Autodesk Inventor part; units mm, degrees
ref_plane "YZ Plane" through (0, 0, 0) normal (1, 0, 0) x (0, 1, 0)
ref_plane "XZ Plane" through (0, 0, 0) normal (0, 1, 0) x (-1, 0, 0)
ref_plane "XY Plane" through (0, 0, 0) normal (0, 0, 1) x (1, 0, 0)
sketch "Skizze1" plane through (0, 0, 0) normal (0, 1, 0) x (-1, 0, 0)
  line L0 (0, -28.6) -> (0, 10.6)
  line L1 (-14, 0) -> (14, 0)
  line L2 (-10, 5) -> (10, 5)
  line L3 (10, 5) -> (10, -5)
  line L4 (10, -5) -> (-10, -5)
  line L5 (-10, -5) -> (-10, 5)
  line L6 (-10, 5) -> (10, -5) construction
  line L7 (10, 5) -> (-10, -5) construction
  line L8 (-5, -5) -> (5, -5)
  line L9 (5, -5) -> (5, -23)
  line L10 (5, -23) -> (-5, -23)
  line L11 (-5, -23) -> (-5, -5)
  line L12 (-5, -5) -> (5, -23) construction
  line L13 (5, -5) -> (-5, -23) construction
  point P0 (0, 0)
  point P1 (0, -14)
  point P2 (-5, -5)
  point P3 (5, -5)
  dimension "d0" = 20
  dimension "d1" = 10
  dimension "d2" = 10
  dimension "d3" = 18
extrude "Extrusion1" add sketch "Skizze1" along normal blind 5
sketch "Skizze2" plane through (0, 5, 0) normal (0, 1, 0) x (1, 0, 0)
  line L0 (0, 28.6) -> (0, -10.6)
  line L1 (5, 23) -> (-5, 23)
  line L2 (-10, -5) -> (10, -5)
  point P0 (0, 0)
  point P1 (0, 17)
  dimension "d14" = 22
hole "Bohrung1" at (0, 5, -17) direction (0, -1, 0) diameter 3.4 end through all counterbore diameter 6.5 counterbore depth 3.4
sketch "Skizze3" plane through (0, 5, 0) normal (0, 1, 0) x (1, 0, 0)
  line L0 (-10, -5) -> (10, -5)
  line L1 (10, -5) -> (10, 5)
  line L2 (-10, -5) -> (10, -5)
  line L3 (10, -5) -> (10, 5)
  line L4 (10, 5) -> (-10, 5)
  line L5 (-10, 5) -> (-10, -5)
  point P0 (0, 0)
extrude "Extrusion2" add sketch "Skizze3" along normal blind 2
sketch "Skizze4" plane through (0, 0, 0) normal (0, -1, 0) x (1, 0, 0)
  line L0 (-10, 5) -> (10, 5)
  line L1 (10, -5) -> (5, -5)
  line L2 (10, 5) -> (7.75, 5)
  line L3 (7.75, 5) -> (7.75, -5)
  line L4 (7.75, -5) -> (10, -5)
  line L5 (10, -5) -> (10, 5)
  point P0 (0, 0)
  dimension "d17" = 2.25
extrude "Extrusion3" add sketch "Skizze4" along normal blind 2
mirror "Spiegeln1" about plane through (0, 0, 0) normal (1, 0, 0) of "Extrusion3"
fillet "Rundung1" radius 2 4 edges at (5, 2.5, -23) (-5, 2.5, -23) (10, 2.5, 5) (-10, 2.5, 5)
fillet "Rundung2" radius 2 2 edges at (10, 2.5, -5) (-10, 2.5, -5)
properties part number "28_Switch_Holder_Y" material "PET-Kunststoff"
Check sheet for the modelled part. Datum: model origin and axes. Units: mm. A direction names the side the tool comes from. Round coordinates to 2 decimals unless told otherwise and drop trailing zeros. Loops run counter-clockwise (first coordinate to the right, second up) from the corner with the lowest first, then second, coordinate; pieces in that order, holes last.
1. Sectioned sample at B-B on x = 0. Record the boundary of the cut face in (y, z).
2. Scan lines: probe 1 along X at (y, z) = (4, -17); probe 2 along Z at (x, y) = (0, 2.9); probe 3 along X at (y, z) = (0.85, -17). Record each from-to range of solid material in increasing order.
3. Gauge pin test, flat ends, axial feed: pin 1 Ø8 at (x, z) = (-1.5, -6) entering from -Y; pin 2 Ø3 at (x, z) = (6, -17) entering from +Y; pin 3 Ø1 at (x, z) = (-1.5, -17) entering from +Y. Record the tip position at first contact, or that the pin passes through.
4. Set-up check for faces 1 (the flat face through (1.4, 1.6, -15.6)), 2 (the flat face through (7.75, -1, 0)), 3 (the flat face through (0, 5, -12)), 4 (the flat face through (5, 2, -13)): record each of +Z, -Z, +X, -X, +Y, -Y from which the full face is reachable in a straight line by a thin tool's end or side.
5. Sectioned sample at C-C on z = -17. Record the boundary of the cut face in (x, y), and give its area (3 significant figures).
6. Sectioned sample at D-D on y = -1. Record the boundary of the cut face in (x, z), and give its area (3 significant figures).
7. Sectioned sample at A-A on y = 3.75. Record the boundary of the cut face in (x, z).
Recorded:
1. outline: (0, -23) - (5, -23) - (5, -20.25) - (1.6, -20.25) - (1.6, -18.7) - (0, -18.7) - close; (0, -15.3) - (1.6, -15.3) - (1.6, -13.75) - (5, -13.75) - (5, -5) - (7, -5) - (7, 5) - (0, 5) - close
2. probe 1: x = -5 to -3.25, 3.25 to 5
2. probe 2: z = -23 to -20.25, -13.75 to 5
2. probe 3: x = -5 to -1.7, 1.7 to 5
3. pin 1: stops at y = 0
3. pin 2: stops at y = 5
3. pin 3: stops at y = 1.6
4. face 1: +Y
4. face 2: +Z, -Z, -Y
4. face 3: -Z, +X, -X, +Y
4. face 4: -Z, +X, +Y, -Y
5. outline: (-5, 0) - (-1.7, 0) - (-1.7, 1.6) - (-3.25, 1.6) - (-3.25, 5) - (-5, 5) - close; (1.7, 0) - (5, 0) - (5, 5) - (3.25, 5) - (3.25, 1.6) - (1.7, 1.6) - close
5. area: 22.5 mm2
6. outline: (-10, -3) arc R2 ccw to (-8, -5) - (-7.75, -5) - (-7.75, 5) - (-8, 5) arc R2 ccw to (-10, 3) - close; (7.75, -5) - (8, -5) arc R2 ccw to (10, -3) - (10, 3) arc R2 ccw to (8, 5) - (7.75, 5) - close
6. area: 41.6 mm2
7. outline: (-10, -3) arc R2 ccw to (-8, -5) - (-5, -5) - (-5, -21) arc R2 ccw to (-3, -23) - (3, -23) arc R2 ccw to (5, -21) - (5, -5) - (8, -5) arc R2 ccw to (10, -3) - (10, 3) arc R2 ccw to (8, 5) - (-8, 5) arc R2 ccw to (-10, 3) - close; hole circle Ø6.5 at (0, -17)
